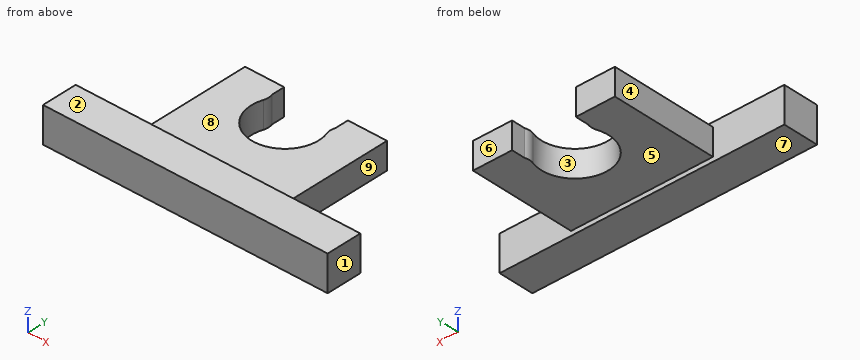
Autodesk Inventor part; units mm, degrees
ref_plane "YZ Plane" through (0, 0, 0) normal (1, 0, 0) x (0, 1, 0)
ref_plane "XZ Plane" through (0, 0, 0) normal (0, 1, 0) x (-1, 0, 0)
ref_plane "XY Plane" through (0, 0, 0) normal (0, 0, 1) x (1, 0, 0)
sketch "Sketch1" plane through (0, 0, 0) normal (0, 1, 0) x (-1, 0, 0)
  line L0 (0, 0) -> (-160.48, 0)
  line L1 (-160.48, 0) -> (-160.48, -20)
  line L2 (-160.48, -20) -> (0, -20)
  line L3 (0, -20) -> (0, 0)
  dimension "d0" = 160.48
  dimension "d1" = 20
extrude "Extrusion1" add sketch "Sketch1" along normal blind 20
sketch "Sketch2" plane through (0, 20, 0) normal (0, 1, 0) x (1, 0, 0)
  line L0 (40.24, 17.5) -> (120.24, 17.5)
  line L1 (120.24, 17.5) -> (120.24, 2.5)
  line L2 (120.24, 2.5) -> (40.24, 2.5)
  line L3 (40.24, 2.5) -> (40.24, 17.5)
  line L4 (160.48, 20) -> (0, 20)
  line L5 (160.48, 0) -> (160.48, 20)
  point P0 (0, 0)
  point P1 (80.24, 17.5)
  point P2 (80.24, 20)
  point P3 (160.48, 10)
  point P4 (120.24, 10)
  dimension "d4" = 80
  dimension "d5" = 15
extrude "Extrusion2" add sketch "Sketch2" along normal blind 60
sketch "Sketch3" plane through (40.24, 20, -2.5) normal (0, 0, 1) x (1, 0, 0)
  circle A0 centre (40, 41) radius 19
  line L0 (0, 60) -> (80, 60)
  point P0 (-40.24, -20)
  point P1 (40, 60)
  dimension "d8" = 38
  dimension "d9" = 19
extrude "Extrusion3" cut sketch "Sketch3" against normal blind 15
sketch "Sketch4" plane through (40.24, 20, -2.5) normal (0, 0, 1) x (1, 0, 0)
  line L0 (22.0399, 60) -> (22.0399, 52.4283)
  line L1 (22.0399, 52.4283) -> (24.8213, 52.4283)
  circle A0 centre (40, 41) radius 19
  line L2 (40, 60) -> (22.0399, 60)
  arc A1 (40, 60) -> (24.8213, 52.4283) centre (40, 41) ccw
  point P0 (-40.24, -20)
  dimension "d12" = 7.5717
  dimension "d13" = 17.9601
extrude "Extrusion4" cut sketch "Sketch4" against normal blind 15 contours L2 A0 L1 L0
sketch "Sketch5" plane through (40.24, 20, -2.5) normal (0, 0, 1) x (1, 0, 0)
  arc A0 (24.8213, 52.4283) -> (40, 60) centre (40, 41) ccw
  line L0 (55.1787, 52.4283) -> (57.9578, 52.4283)
  line L1 (57.9578, 52.4283) -> (57.9578, 60)
  line L2 (57.9578, 60) -> (40, 60)
  line L3 (80, 60) -> (40, 60)
  arc A1 (55.1787, 52.4283) -> (40, 60) centre (40, 41) ccw
  point P0 (-40.24, -20)
  dimension "d16" = 17.9578
  dimension "d17" = 2.7791
  dimension "d18" = 7.5717
extrude "Extrusion5" cut sketch "Sketch5" against normal blind 15
fillet "Fillet1" radius 7.62 1 edges at (95.4187, 72.4283, -10)
fillet "Fillet2" radius 7.62 1 edges at (65.0613, 72.4283, -10)
properties part number "OpticalDeviceLensHolder"
Part model, mm, in its own coordinate system. Face numbers are marked on the shaded views. A direction names the side the tool comes from. Round coordinates to 2 decimals unless told otherwise and drop trailing zeros. Write each loop counter-clockwise with the first axis right and the second up, starting at its lowest first coordinate (ties: lowest second). Pieces come first, ordered by that corner, then holes.
Item 1: Cut at D-D, the plane y = 25.5. Give the cut face in (x, z), plus the area to 3 significant figures.
Results:
outline: (40.24, -17.5) - (120.24, -17.5) - (120.24, -2.5) - (40.24, -2.5) - close
area: 1,200 mm2
Item 2: Cut at A-A, the plane y = 61. Give the cut face in (x, z), plus the area to 3 significant figures.
Results:
outline: (40.24, -17.5) - (61.24, -17.5) - (61.24, -2.5) - (40.24, -2.5) - close; (99.24, -17.5) - (120.24, -17.5) - (120.24, -2.5) - (99.24, -2.5) - close
area: 630 mm2
Item 3: Two-plate mould, pull along X, no slides. Class the marked faces 1, 2, 3 and 4: +X half, -X half, draft (parallel to the pull), parting line (faces both ways), or undercut.
Results:
face 1: +X half
face 2: draft
face 3: undercut
face 4: -X half
Item 4: Which spindle directions (+Z, -Z, +X, -X, +Y, -Y) get a long thin tool onto all of the face, cutting with end or side? Do the marked faces 5, 6, 7, 8 and 9. Say none if no direction does.
Results:
face 5: -Z, +X, -X, +Y
face 6: +Z, -Z, +X, -X, +Y
face 7: -Z, +X, -X, +Y, -Y
face 8: +Z, +X, -X, +Y
face 9: +Z, -Z, +X, +Y
Item 5: Cut at C-C, the plane z = -4.25. Give the cut face in (x, y), plus the area to 3 significant figures.
Results:
outline: (0, 0) - (160.48, 0) - (160.48, 20) - (120.24, 20) - (120.24, 80) - (98.2, 80) - (98.2, 72.43) arc R7.62 ccw to (98.17, 67.29) arc R19 cw (long way) to (62.31, 67.29) arc R7.62 ccw to (62.28, 72.43) - (62.28, 80) - (40.24, 80) - (40.24, 20) - (0, 20) - close
area: 6,750 mm2
Item 6: Probe L1, parallel to X at y = 61, z = -9; L2, parallel to Y at x = 19.5, z = -18.5; L3, parallel to Z at x = 79, y = 34. List the from-to ranges inside material, lowest first.
Results:
L1: x = 40.24 to 61.24, 99.24 to 120.24
L2: y = 0 to 20
L3: z = -17.5 to -2.5
Item 7: Cut at B-B, the plane x = 80.24. Give the cut face in (y, z).
Results:
outline: (0, -20) - (20, -20) - (20, -17.5) - (42, -17.5) - (42, -2.5) - (20, -2.5) - (20, 0) - (0, 0) - close
Item 8: Drop flat-ended pins along their axis: pin 1 Ø3 at (y, z) = (24, -4) entering from -X; pin 2 Ø2 at (x, z) = (96.5, -13.5) entering from +Y; pin 3 Ø6 at (x, y) = (42.5, 39) entering from +Z. Give the stop position or say it passes through.
Results:
pin 1: stops at x = 40.24
pin 2: stops at y = 53.06
pin 3: stops at z = -2.5
